Here's how the part is built. I have some questions about the finished solid (model axes, mm). A direction names the side the tool comes from. Round coordinates to 2 decimals unless told otherwise and drop trailing zeros. Order: outer loops, then holes, each group sorted by start corner. A loop starts at its lowest first (then second) coordinate and runs counter-clockwise, first axis right, second up. Notation, with made-up numbers: (23.5, 89.25) -> (46.5, 89.25) arc R21 ccw to (46.5, 105.25) -> close; hole circle Ø3 at (49, 9.25). An arc over 180 degrees is marked (long way). Answer in a Markdown table with one row per item.
```python
from build123d import *

# Parameters (mm, degrees)
SKETCH1_W           = 18
SKETCH1_H           = 58
BOSS_EXTRUDE1_DEPTH = 3.5
SKETCH2_W           = 17
SKETCH2_H           = 7
CUT_EXTRUDE1_DEPTH  = 5
CHAMFER1_SIZE2      = 3
CHAMFER1_SIZE       = 7
FILLET2_R           = 1
SKETCH3_W           = 8.5
SKETCH3_H           = 3.471291158
BOSS_EXTRUDE2_DEPTH = 0.1


# Some blends are built 0.0001 mm under size
with BuildPart() as part:
    # Sketch1 → Boss-Extrude1 (new, symmetric)
    with BuildSketch(Plane(origin=(0, 0, 0), x_dir=(1, 0, 0), z_dir=(0, 1, 0))):
        Rectangle(SKETCH1_W, SKETCH1_H)
    extrude(amount=BOSS_EXTRUDE1_DEPTH, both=True)

    # Sketch2 → Cut-Extrude1 (cut)
    with BuildSketch(Plane.XZ.offset(3.5)):
        with Locations((0, 25.5)):
            Rectangle(SKETCH2_W, SKETCH2_H)
    extrude(amount=-CUT_EXTRUDE1_DEPTH, mode=Mode.SUBTRACT)

    # Chamfer1
    chamfer1_edges = [part.edges().sort_by_distance(p)[0] for p in [
        (0, 1.5, 22),
    ]]
    chamfer1_side = [part.faces().sort_by_distance(p)[0] for p in [
        (0, 1.5, 22.06),
    ]]
    chamfer(chamfer1_edges, length=CHAMFER1_SIZE - 0.0001, length2=CHAMFER1_SIZE2 - 0.0001, reference=chamfer1_side[0])  # a hair under: the kernel refuses the full size

    # Fillet2
    # the kernel refuses this fillet: 1 mm, written as the material it takes off along each edge
    with BuildSketch(Plane(origin=(8, -2.5, -28), x_dir=(1, 0, 0), z_dir=(0, 0, -1))) as fillet2_piece_1_section:
        Polygon((0, 0), (FILLET2_R, 0), (FILLET2_R, FILLET2_R), (0, FILLET2_R), align=None)
    fillet2_piece_1 = extrude(amount=FILLET2_R, mode=Mode.PRIVATE)
    fillet2_piece_1 = fillet2_piece_1 - Plane(origin=(8, -2.5, -28), x_dir=(-0.7071067811865475, 0.7071067811865475, 0), z_dir=(0, 0, -1)) * Sphere(FILLET2_R, mode=Mode.PRIVATE)
    add(fillet2_piece_1, mode=Mode.SUBTRACT)
    with BuildSketch(Plane(origin=(-8, -2.5, -28), x_dir=(0, -1, 0), z_dir=(0, 0, -1))) as fillet2_piece_2_section:
        Polygon((0, 0), (FILLET2_R, 0), (FILLET2_R, FILLET2_R), (0, FILLET2_R), align=None)
    fillet2_piece_2 = extrude(amount=FILLET2_R, mode=Mode.PRIVATE)
    fillet2_piece_2 = fillet2_piece_2 - Plane(origin=(-8, -2.5, -28), x_dir=(0.7071067811865475, 0.7071067811865475, 0), z_dir=(0, 0, -1)) * Sphere(FILLET2_R, mode=Mode.PRIVATE)
    add(fillet2_piece_2, mode=Mode.SUBTRACT)
    with BuildSketch(Plane(origin=(-8, 2.5, -28), x_dir=(0, 1, 0), z_dir=(0, 0, -1))) as fillet2_piece_3_section:
        Polygon((0, 0), (FILLET2_R, 0), (FILLET2_R, -FILLET2_R), (0, -FILLET2_R), align=None)
    fillet2_piece_3 = extrude(amount=FILLET2_R, mode=Mode.PRIVATE)
    fillet2_piece_3 = fillet2_piece_3 - Plane(origin=(-8, 2.5, -28), x_dir=(0.7071067811865475, -0.7071067811865475, 0), z_dir=(0, 0, -1)) * Sphere(FILLET2_R, mode=Mode.PRIVATE)
    add(fillet2_piece_3, mode=Mode.SUBTRACT)
    with BuildSketch(Plane(origin=(8, 2.5, -28), x_dir=(1, 0, 0), z_dir=(0, 0, -1))) as fillet2_piece_4_section:
        Polygon((0, 0), (FILLET2_R, 0), (FILLET2_R, -FILLET2_R), (0, -FILLET2_R), align=None)
    fillet2_piece_4 = extrude(amount=FILLET2_R, mode=Mode.PRIVATE)
    fillet2_piece_4 = fillet2_piece_4 - Plane(origin=(8, 2.5, -28), x_dir=(-0.7071067811865475, -0.7071067811865475, 0), z_dir=(0, 0, -1)) * Sphere(FILLET2_R, mode=Mode.PRIVATE)
    add(fillet2_piece_4, mode=Mode.SUBTRACT)
    with BuildSketch(Plane(origin=(-8, 2.5, 28), x_dir=(0, 0, 1), z_dir=(0, 1, 0))) as fillet2_piece_5_section:
        Polygon((0, 0), (FILLET2_R, 0), (FILLET2_R, -FILLET2_R), (0, -FILLET2_R), align=None)
    fillet2_piece_5 = extrude(amount=FILLET2_R, mode=Mode.PRIVATE)
    fillet2_piece_5 = fillet2_piece_5 - Plane(origin=(-8, 2.5, 28), x_dir=(0.7071067811865475, 0, -0.7071067811865475), z_dir=(0, 1, 0)) * Sphere(FILLET2_R, mode=Mode.PRIVATE)
    add(fillet2_piece_5, mode=Mode.SUBTRACT)
    with BuildSketch(Plane(origin=(8, 2.5, 28), x_dir=(0, 1, 0), z_dir=(1, 0, 0))) as fillet2_piece_6_section:
        Polygon((0, 0), (FILLET2_R, 0), (FILLET2_R, FILLET2_R), (0, FILLET2_R), align=None)
    fillet2_piece_6 = extrude(amount=FILLET2_R, mode=Mode.PRIVATE)
    fillet2_piece_6 = fillet2_piece_6 - Plane(origin=(8, 2.5, 28), x_dir=(0, -0.7071067811865475, -0.7071067811865475), z_dir=(1, 0, 0)) * Sphere(FILLET2_R, mode=Mode.PRIVATE)
    add(fillet2_piece_6, mode=Mode.SUBTRACT)
    with BuildSketch(Plane(origin=(8, -3.5, -29), x_dir=(0, 0, 1), z_dir=(-1, 0, 0)), Plane(origin=(8, 3.5, -29), x_dir=(0, -1, 0), z_dir=(-1, 0, 0)), Plane(origin=(-8, 3.5, 29), x_dir=(0, -1, 0), z_dir=(1, 0, 0))) as fillet2_piece_7:
        with BuildLine():
            CenterArc((FILLET2_R, FILLET2_R), FILLET2_R, 180, 90)
            Line((0, FILLET2_R), (0, 0))
            Line((0, 0), (FILLET2_R, 0))
        make_face()
    extrude(amount=16, mode=Mode.SUBTRACT)
    with BuildSketch(Plane(origin=(-9, 2.5, -29), x_dir=(0, 0, 1), z_dir=(0, -1, 0))) as fillet2_piece_8:
        with BuildLine():
            CenterArc((FILLET2_R, -FILLET2_R), FILLET2_R, 90, 90)
            Line((0, -FILLET2_R), (0, 0))
            Line((0, 0), (FILLET2_R, 0))
        make_face()
    extrude(amount=5, mode=Mode.SUBTRACT)
    with BuildSketch(Plane(origin=(-9, -3.5, -28), x_dir=(1, 0, 0), z_dir=(0, 0, 1)), Plane(origin=(9, -3.5, 31.5), x_dir=(-1, 0, 0), z_dir=(0, 0, -1))) as fillet2_piece_9:
        with BuildLine():
            CenterArc((FILLET2_R, FILLET2_R), FILLET2_R, 180, 90)
            Line((0, FILLET2_R), (0, 0))
            Line((0, 0), (FILLET2_R, 0))
        make_face()
    extrude(amount=59.5, mode=Mode.SUBTRACT)
    with BuildSketch(Plane(origin=(-9, 3.5, -28), x_dir=(0, -1, 0), z_dir=(0, 0, 1)), Plane(origin=(9, 3.5, 28), x_dir=(0, -1, 0), z_dir=(0, 0, -1))) as fillet2_piece_10:
        with BuildLine():
            CenterArc((FILLET2_R, FILLET2_R), FILLET2_R, 180, 90)
            Line((0, FILLET2_R), (0, 0))
            Line((0, 0), (FILLET2_R, 0))
        make_face()
    extrude(amount=56, mode=Mode.SUBTRACT)
    with BuildSketch(Plane(origin=(9, -2.5, -29), x_dir=(-1, 0, 0), z_dir=(0, 1, 0))) as fillet2_piece_11:
        with BuildLine():
            CenterArc((FILLET2_R, FILLET2_R), FILLET2_R, 180, 90)
            Line((0, FILLET2_R), (0, 0))
            Line((0, 0), (FILLET2_R, 0))
        make_face()
    extrude(amount=5, mode=Mode.SUBTRACT)
    with BuildSketch(Plane(origin=(-9, 2.5, 29), x_dir=(1, 0, 0), z_dir=(0, -1, 0)), Plane(origin=(9, -6, 29), x_dir=(-1, 0, 0), z_dir=(0, 1, 0))) as fillet2_piece_12:
        with BuildLine():
            CenterArc((FILLET2_R, -FILLET2_R), FILLET2_R, 90, 90)
            Line((0, -FILLET2_R), (0, 0))
            Line((0, 0), (FILLET2_R, 0))
        make_face()
    extrude(amount=8.5, mode=Mode.SUBTRACT)

    # Sketch3 → Boss-Extrude2 (add)
    with BuildSketch(Plane.XY.offset(22)):
        with Locations((-4.25, -1.764354421)):
            Rectangle(SKETCH3_W, SKETCH3_H)
    extrude(amount=BOSS_EXTRUDE2_DEPTH)


solid = part.part
```
1. Suppose I cut it at B-B on y = 0.25. Write out the boundary of the cut face in (x, z).
Numbers:
| item | result |
|---|---|
| outline | (-9, -28) arc R1 ccw to (-8, -29) -> (8, -29) arc R1 ccw to (9, -28) -> (9, 28) arc R1 ccw to (8.5, 28.87) -> (8.5, 26.08) -> (-8.5, 26.08) -> (-8.5, 28.87) arc R1 ccw to (-9, 28) -> close |
2. For faces 4 (the face through (-8.5, -2, 26)), 5 (the face through (0, 0, -29)), which set-ups out of +Z, -Z, +X, -X, +Y, -Y let a thin tool reach every point of the face, with its end or its side?
Numbers:
| item | result |
|---|---|
| face 4 | +Z, -Y |
| face 5 | -Z, +X, -X, +Y, -Y |
3. Please list where these lines run through material, in increasing order: line 1 along Z through (x, y) = (-5.5, -2.5); line 2 along Z through (x, y) = (1.5, -1.75); line 3 along X through (y, z) = (3.25, 6).
Numbers:
| item | result |
|---|---|
| line 1 | z = -29 to 22.1 |
| line 2 | z = -29 to 22 |
| line 3 | x = -8.66 to 8.66 |
4. We'd pull the mould along X, two halves only. Please class faces 1 (the face through (4, -3, 22)), 2 (the face through (-8.8, 0.3, 28.6)), 3 (the face through (0, -3.5, -3)): released by +X, released by -X, zero draft, split by the parting line, or undercut.
Numbers:
| item | result |
|---|---|
| face 1 | undercut |
| face 2 | released by -X |
| face 3 | zero draft |
5. For pin 1 Ø0.6 at (x, y) = (4, -2.5) entering from +Z; pin 2 Ø2 at (x, y) = (-2.5, -2) entering from +Z, each with a flat end and sliding along its axis, tell me the tip position at first contact or that it passes through.
Numbers:
| item | result |
|---|---|
| pin 1 | stops at z = 22 |
| pin 2 | stops at z = 23.17 |
